Check sheet for the modelled part. Datum: model origin and axes. Units: mm. A direction names the side the tool comes from. Round coordinates to 2 decimals unless told otherwise and drop trailing zeros. Write each loop counter-clockwise with the first axis right and the second up, starting at its lowest first coordinate (ties: lowest second). Pieces come first, ordered by that corner, then holes. Notation, with made-up numbers: (33.5, 12) -> (59.5, 12) arc R12 ccw to (59.5, 30) -> close; hole circle Ø1 at (-24.5, -0.75). An arc over 180 degrees is marked (long way). One line per item, written item: value.
Autodesk Inventor part; units mm, degrees
ref_plane "YZ Plane" through (0, 0, 0) normal (1, 0, 0) x (0, 1, 0)
ref_plane "XZ Plane" through (0, 0, 0) normal (0, 1, 0) x (-1, 0, 0)
ref_plane "XY Plane" through (0, 0, 0) normal (0, 0, 1) x (1, 0, 0)
sketch "Sketch4" plane through (0, 0, 0) normal (0, 1, 0) x (-1, 0, 0)
  circle A0 centre (0, 0) radius 17.5
extrude "Extrusion2" add sketch "Sketch4" along normal mid plane 12
sketch "Sketch12" plane through (0, 6, 0) normal (0, 1, 0) x (1, 0, 0)
  circle A0 centre (0, 0) radius 16.5
  dimension "d85" = 33
extrude "Extrusion8" cut sketch "Sketch12" against normal blind 10
sketch "Sketch13" plane through (0, -4, 0) normal (0, 1, 0) x (1, 0, 0)
  point P0 (0, 0)
chamfer "Chamfer1" distance 0.2 angle 45 3 edges at (17.5, 6, 0) (-16.5, 6, 0) (17.5, -6, 0)
properties part number "Shallow Dish" material "Brass, Soft Yellow"
Item 1: Sectioned sample at C-C on y = -1.5. Enter the section's corners in (x, z), and give its area (3 significant figures).
Answer:
outline: circle Ø35 at (0, 0); hole circle Ø33 at (0, 0)
area: 107 mm^2
Item 2: Thickness scan on line 1 (Z direction, x = 0, y = 3.5); line 2 (Y direction, x = -10.5, z = -9); line 3 (X direction, y = -3, z = 6.5). Record the ranges inside material, lowest first.
Answer:
line 1: z = -17.5 to -16.5, 16.5 to 17.5
line 2: y = -6 to -4
line 3: x = -16.25 to -15.17, 15.17 to 16.25
Item 3: Tool access check on faces 1 (the flat face through (0, -6, 0)), 2 (the cylindrical face through (15.24, 0.97, 6.32)). Record the directions out of +Z, -Z, +X, -X, +Y, -Y that give a thin tool (end or side, any length) a straight path to the whole face; none if there is none.
Answer:
face 1: +Z, -Z, +X, -X, -Y
face 2: +Y
Item 4: Sectioned sample at A-A on z = 0. Enter the section's corners in (x, y), and give its area (3 significant figures).
Answer:
outline: (-17.5, -5.8) -> (-17.3, -6) -> (17.3, -6) -> (17.5, -5.8) -> (17.5, 5.8) -> (17.3, 6) -> (16.7, 6) -> (16.5, 5.8) -> (16.5, -4) -> (-16.5, -4) -> (-16.5, 5.8) -> (-16.7, 6) -> (-17.3, 6) -> (-17.5, 5.8) -> close
area: 89.9 mm^2
Item 5: Sectioned sample at D-D on y = -5. Enter the section's corners in (x, z).
Answer:
outline: circle Ø35 at (0, 0)
Item 6: Sectioned sample at B-B on x = 0. Enter the section's corners in (y, z).
Answer:
outline: (-6, -17.3) -> (-5.8, -17.5) -> (5.8, -17.5) -> (6, -17.3) -> (6, -16.7) -> (5.8, -16.5) -> (-4, -16.5) -> (-4, 16.5) -> (5.8, 16.5) -> (6, 16.7) -> (6, 17.3) -> (5.8, 17.5) -> (-5.8, 17.5) -> (-6, 17.3) -> close
Item 7: Depth check by flat-ended pin: P1, Ø5, axis at x = -9.5, z = -10.5, coming from the +Y side; P2, Ø4, axis at y = -2.5, z = -2.5, coming from the -X side; P3, Ø3, axis at y = -1, z = 3, coming from the +X side; P4, Ø6, axis at y = 4, z = 1, coming from the +X side. Enter the tip coordinate at first touch or a pass-through.
Answer:
P1: stops at y = 5.96
P2: stops at x = -17.49
P3: stops at x = 17.44
P4: stops at x = 17.5
Item 8: Mould release check, pull along X, two halves, no side actions. Record for faces 3 (the flat face through (9.1, 6, 14.2)), 4 (the cylindrical face through (13.887, -0.081, 10.648)), 5 (the flat face through (0, -4, 0)): pulls with the +X half, pulls with the -X half, needs draft (parallel to the pull), parting line crosses it, or undercut.
Answer:
face 3: needs draft
face 4: parting line crosses it
face 5: undercut
